```python
from build123d import *

# Parameters (mm, degrees)
ESQUISSE1_R                  = 9
BOSS_EXTRU_1_DEPTH           = 2.5
ENL_V_MAT_EXTRU_1_REACH      = 24.773
ENL_V_MAT_EXTRU_1_END_RADIUS = 9
ESQUISSE2_R                  = 0.75
CONG_1_R                     = 1.5
CONG_2_R                     = 0.25


with BuildPart() as part:
    # Esquisse1 → Boss.-Extru.1 (new body)
    with BuildSketch(Plane(origin=(0, 0, 0), x_dir=(1, 0, 0), z_dir=(0, 1, 0))):
        with BuildLine():
            Line((7.806247498, 6.25), (10.306247498, 6.25))
            Line((10.306247498, 6.25), (10.306247498, -6.25))
            Line((10.306247498, -6.25), (7.806247498, -6.25))
            ThreePointArc((7.806247498, -6.25), (-10, 0), (7.806247498, 6.25))
        make_face()
        with Locations(Location((0, 0, 0), (0, 0, 270))):
            Circle(ESQUISSE1_R, mode=Mode.SUBTRACT)
    extrude(amount=BOSS_EXTRU_1_DEPTH)

    # Enlèv. mat.-Extru.1: up to this cylinder (the profile starts outside it)
    enl_v_mat_extru_1_end = Plane(origin=(0, 1.25, 0), z_dir=(0, -1, 0)) * Cylinder(ENL_V_MAT_EXTRU_1_END_RADIUS, 68.546, mode=Mode.PRIVATE)
    # Esquisse2 → Enlèv. mat.-Extru.1 (cut, up to the surface)
    with BuildSketch(Plane(origin=(10.306247498, 0, 0), x_dir=(0, 0, -1), z_dir=(1, 0, 0)), mode=Mode.PRIVATE) as enl_v_mat_extru_1_sk1:
        with Locations((0, 1.25)):
            Circle(ESQUISSE2_R)
    enl_v_mat_extru_1_tool1 = extrude(enl_v_mat_extru_1_sk1.sketch, amount=-ENL_V_MAT_EXTRU_1_REACH, mode=Mode.PRIVATE) - enl_v_mat_extru_1_end
    add(enl_v_mat_extru_1_tool1.solids().sort_by_distance((10.306247, 1.25, 0))[0], mode=Mode.SUBTRACT)

    # Congé1
    cong_1_edges = [part.edges().sort_by_distance(p)[0] for p in [
        (7.806247498, 1.25, -6.25),
        (10.306247498, 1.25, -6.25),
        (10.306247498, 1.25, 6.25),
        (7.806247498, 1.25, 6.25),
    ]]
    fillet(cong_1_edges, radius=CONG_1_R)

    # Congé2
    cong_2_edges = [part.edges().sort_by_distance(p)[0] for p in [
        (0, 0, -9),
        (0, 2.5, -9),
        (10.306247498, 0, 0),
        (10.306247498, 2.5, 0),
        (-10, 0, 0),
        (8.651285116, 0, -6.25),
        (8.651285116, 0, 6.25),
        (9.86690767, 0, -5.810660172),
        (9.86690767, 0, 5.810660172),
        (8.651285116, 2.5, 6.25),
        (-10, 2.5, 0),
        (8.651285116, 2.5, -6.25),
        (9.86690767, 2.5, -5.810660172),
        (9.86690767, 2.5, 5.810660172),
        (7.890643094, 0, 6.377720082),
        (7.890643094, 2.5, 6.377720082),
        (7.890643094, 0, -6.377720082),
        (7.890643094, 2.5, -6.377720082),
    ]]
    fillet(cong_2_edges, radius=CONG_2_R)


solid = part.part
```
Design review of the part built by this model. Coordinates are the model's own, in mm. Coordinates: 2 decimals unless noted, no trailing zeros. Order: outer loops, then holes, each group sorted by start corner. A loop starts at its lowest first (then second) coordinate and runs counter-clockwise, first axis right, second up. Notation, with made-up numbers: (2, 41) -> (38, 41) arc R29 ccw to (38, 68) -> close; hole circle Ø4 at (76, 61.25). An arc over 180 degrees is marked (long way). One line per item, written item: value. Start each with the question number.
Q1. Mouldability with a two-part tool opening along Y and no side actions: class faces 1 (the cylindrical face through (9.647, 0.518, 0.163)), 2 (the flat face through (9, 2.5, 3)), 3 (the cylindrical face through (9.88, 1.26, 5.8)) as pulls with the +Y half, pulls with the -Y half, needs draft (parallel to the pull), parting line crosses it, or undercut.
Q2. Take a section at B-B, the plane y = 1.25. State the section outline as (x, z) points.
Q3. Take a section at A-A, the plane z = 0. State the section outline as (x, y) points, then the cut area to 3 significant figures.
Q4. For probe 1 along Y at (x, z) = (10.05, 0); probe 2 along X at (y, z) = (1.5, -6); probe 3 along Y at (x, z) = (9, -2), list the stretches that pass through material, from the lowest coordinate up.
Values follow:
1. face 1: undercut
1. face 2: pulls with the +Y half
1. face 3: needs draft
2. outline: (7.39, -6.74) arc R1.5 cw to (8.5, -6.25) -> (8.81, -6.25) arc R1.5 ccw to (10.31, -4.75) -> (10.31, -0.75) -> (8.97, -0.75) arc R9 cw (long way) to (8.97, 0.75) -> (10.31, 0.75) -> (10.31, 4.75) arc R1.5 ccw to (8.81, 6.25) -> (8.5, 6.25) arc R1.5 cw to (7.39, 6.74) arc R10 ccw (long way) to start
3. outline: (-10, 0.25) arc R0.25 ccw to (-9.75, 0) -> (-9.25, 0) arc R0.25 ccw to (-9, 0.25) -> (-9, 2.25) arc R0.25 ccw to (-9.25, 2.5) -> (-9.75, 2.5) arc R0.25 ccw to (-10, 2.25) -> close; (9, 0.25) arc R0.25 ccw to (9.25, 0) -> (10.06, 0) arc R0.25 ccw to (10.31, 0.25) -> (10.31, 0.5) -> (9, 0.5) -> close; (9, 2) -> (10.31, 2) -> (10.31, 2.25) arc R0.25 ccw to (10.06, 2.5) -> (9.25, 2.5) arc R0.25 ccw to (9, 2.25) -> close
3. area: 3.70 mm2
4. probe 1: y = 0 to 0.5, 2 to 2.5
4. probe 2: x = -8 to -6.71, 6.71 to 9.64
4. probe 3: y = 0 to 2.5
